Read the model definition and answer for the solid it produces. Units are mm, in the model's axes. A direction names the side the tool comes from. Coordinates: 2 decimals unless noted, no trailing zeros. Write each loop counter-clockwise with the first axis right and the second up, starting at its lowest first coordinate (ties: lowest second). Pieces come first, ordered by that corner, then holes.
(1) The part is cut by section B-B, the plane z = -44.45. Determine the outline of the cut face in (x, y) (1 decimal).
(2) Which of the six approach directions +Z, -Z, +X, -X, +Y, -Y give full straight-line access (tool end or side, diameter ignored) to faces 4 (the cylindrical face through (-1.93, -3.91, 10.18)), 5 (the flat face through (0, 17.462, -40)), 6 (the flat face through (3, 0, 15))?
(3) Given pin 1 (4 mm diameter, centred on x = 0, z = 12.7, fed in from -Y); pin 2 (5 mm diameter, centred on x = -4, y = 11, fed in from -Z); pin 3 (12.5 mm diameter, centred on x = 5, z = 7, fed in from +Y); pin 4 (4 mm diameter, centred on x = 3, y = 4, fed in from +Z), each flat-ended and moving along its own axis, determine where each tip first touches the part or whether it passes through.
(4) Determine the mould class of faces 1 (the flat face through (0, 25.4, -27)), 2 (the flat face through (12.7, 5, -23)), 3 (the flat face through (0, 13, -31.75)) for opening direction Y: pulls with the +Y half, pulls with the -Y half, needs draft (parallel to the pull), parting line crosses it, or undercut.
(5) Straight lines are drawn through the part: line 1 along X through (y, z) = (-5.75, 12.7) (3 decimals); line 2 along Y through (x, z) = (0.5, -39.5); line 3 along Z through (x, y) = (1.5, 16.5). For each, find the intervals that lie inside material, in ascending order.
(6) The part is cut by section A-A, the plane x = 0. State how many separate pieces and enclosed holes the cut face has, and give its area (3 significant figures).
(7) The part is cut by section C-C, the plane z = 12.7. Determine the outline of the cut face in (x, y) (1 decimal), and give its area (3 significant figures).
```python
from build123d import *

# Parameters (mm, degrees)
BOSS_EXTRUDE1_DEPTH = 12.7
SKETCH2_R           = 3.175
CUT_EXTRUDE1_DEPTH  = 65.699146295


with BuildPart() as part:
    # Sketch1 → Boss-Extrude1 (new, symmetric)
    with BuildSketch(Plane(origin=(0, 0, 0), x_dir=(0, 0, -1), z_dir=(1, 0, 0))):
        Polygon((0, 0), (-25.4, 0), (-25.4, -7.9375), (53.975, -7.9375), (53.975, 7.9375), (31.75, 7.9375), (31.75, 17.4625), (53.975, 17.4625), (53.975, 25.4), (0, 25.4), align=None)
    extrude(amount=BOSS_EXTRUDE1_DEPTH, both=True)

    # Sketch2 → Cut-Extrude1 (cut, through all)
    with BuildSketch(Plane(origin=(0, 25.4, 0), x_dir=(1, 0, 0), z_dir=(0, 1, 0))):
        with Locations(Location((0, 44.45, 0), (0, 0, 270))):
            Circle(SKETCH2_R)
        with Locations(Location((0, -12.7, 0), (0, 0, 270))):
            Circle(SKETCH2_R)
    extrude(amount=-CUT_EXTRUDE1_DEPTH, mode=Mode.SUBTRACT)


solid = part.part
```
Computed:
1. outline: (-12.7, -7.9) - (-3.2, -7.9) - (-3.2, 7.9) - (-12.7, 7.9) - close; (-12.7, 17.5) - (-3.2, 17.5) - (-3.2, 25.4) - (-12.7, 25.4) - close; (3.2, -7.9) - (12.7, -7.9) - (12.7, 7.9) - (3.2, 7.9) - close; (3.2, 17.5) - (12.7, 17.5) - (12.7, 25.4) - (3.2, 25.4) - close
2. face 4: +Y, -Y
2. face 5: -Z, +X, -X
2. face 6: +Z, +X, -X, +Y
3. pin 1: passes through
3. pin 2: stops at z = -31.75
3. pin 3: stops at y = 0
3. pin 4: stops at z = 0
4. face 1: pulls with the +Y half
4. face 2: needs draft
4. face 3: undercut
5. line 1: x = -12.7 to -3.175, 3.175 to 12.7
5. line 2: y = -7.94 to 7.94, 17.46 to 25.4
5. line 3: z = -31.75 to 0
6. separate pieces: 4
6. enclosed holes: 0
6. area: 1,590 mm2
7. outline: (-12.7, -7.9) - (-3.2, -7.9) - (-3.2, 0) - (-12.7, 0) - close; (3.2, -7.9) - (12.7, -7.9) - (12.7, 0) - (3.2, 0) - close
7. area: 151 mm2
